Geometry check sheet. Reference: the model listing, model coordinates, mm. Face numbers are marked on the shaded views. A direction names the side the tool comes from. Coordinates: 2 decimals unless noted, no trailing zeros. Write each loop counter-clockwise with the first axis right and the second up, starting at its lowest first coordinate (ties: lowest second). Pieces come first, ordered by that corner, then holes. Notation, with made-up numbers: (88, 37.5) -> (112, 37.5) arc R27 ccw to (112, 72.5) -> close; hole circle Ø6 at (83.5, 38). An arc over 180 degrees is marked (long way). Use a Markdown table: item, result.
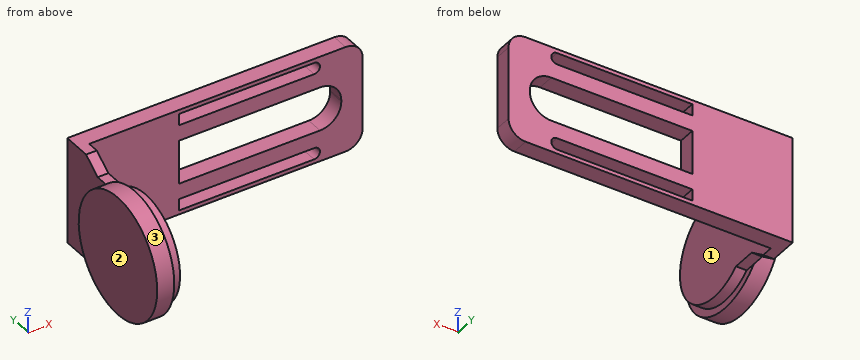
```python
from build123d import *

# Parameters (mm, degrees)
BOSS_EXTRUDE1_DEPTH = 4
BOSS_EXTRUDE2_DEPTH = 2.5
SKETCH3_R           = 14
BOSS_EXTRUDE3_DEPTH = 4


with BuildPart() as part:
    # Sketch1 → Boss-Extrude1 (new body)
    with BuildSketch(Plane(origin=(0, 0, 0), x_dir=(1, 0, 0), z_dir=(0, 1, 0))):
        with BuildLine():
            Line((0, 0), (62.5, 0))
            ThreePointArc((62.5, 0), (65.328427125, -1.171572875), (66.5, -4))
            Line((66.5, -4), (66.5, -21))
            ThreePointArc((66.5, -21), (65.328427125, -23.828427125), (62.5, -25))
            Line((62.5, -25), (0, -25))
            Line((0, -25), (0, 0))
        make_face()
        with BuildLine():
            Line((23.5, -7.35), (56.51, -7.35))
            ThreePointArc((56.51, -7.35), (60.038462838, -8.811537162), (61.5, -12.34))
            Line((61.5, -12.34), (61.5, -12.66))
            ThreePointArc((61.5, -12.66), (60.038462838, -16.188462838), (56.51, -17.65))
            Line((56.51, -17.65), (23.5, -17.65))
            Line((23.5, -17.65), (23.5, -7.35))
        make_face(mode=Mode.SUBTRACT)
        with BuildLine():
            Line((23.5, -0.96), (55.151, -0.96))
            ThreePointArc((55.151, -0.96), (56.104887048, -1.355112952), (56.5, -2.309))
            Line((56.5, -2.309), (56.5, -2.311))
            ThreePointArc((56.5, -2.311), (56.104887048, -3.264887048), (55.151, -3.66))
            Line((55.151, -3.66), (23.5, -3.66))
            Line((23.5, -3.66), (23.5, -0.96))
        make_face(mode=Mode.SUBTRACT)
        with BuildLine():
            Line((23.5, -21.34), (55.151, -21.34))
            ThreePointArc((55.151, -21.34), (56.104887048, -21.735112952), (56.5, -22.689))
            Line((56.5, -22.689), (56.5, -22.691))
            ThreePointArc((56.5, -22.691), (56.104887048, -23.644887048), (55.151, -24.04))
            Line((55.151, -24.04), (23.5, -24.04))
            Line((23.5, -24.04), (23.5, -21.34))
        make_face(mode=Mode.SUBTRACT)
    extrude(amount=BOSS_EXTRUDE1_DEPTH)

    # Sketch2 → Boss-Extrude2 (add)
    with BuildSketch(Plane.ZY):
        with BuildLine():
            Line((3, -6.816145851), (3, -12.416145851))
            ThreePointArc((3, -12.416145851), (12.5, -32.4), (22, -12.416145851))
            Line((22, -12.416145851), (22, -6.816145851))
            Line((22, -6.816145851), (25, -2.7))
            Line((25, -2.7), (25, 0))
            Line((25, 0), (0, 0))
            Line((0, 0), (0, -2.7))
            Line((0, -2.7), (3, -6.816145851))
        make_face()
    extrude(amount=-BOSS_EXTRUDE2_DEPTH)

    # Sketch3 → Boss-Extrude3 (add)
    with BuildSketch(Plane.ZY):
        with Locations(Location((12.5, -20.15, 0), (0, 0, 132.732110043))):
            Circle(SKETCH3_R)
    extrude(amount=BOSS_EXTRUDE3_DEPTH)


solid = part.part
```
Item 1: Section check C-C on y = -20.15. Record the boundary of the cut face in (x, z), then the cut area to 3 significant figures.
Answer block:
| item | result |
|---|---|
| outline | (-4, -1.5) -> (0, -1.5) -> (0, 0.25) -> (2.5, 0.25) -> (2.5, 24.75) -> (0, 24.75) -> (0, 26.5) -> (-4, 26.5) -> close |
| area | 173 mm^2 |
Item 2: Section check D-D on z = 19. Record the boundary of the cut face in (x, y), then the cut area to 3 significant figures.
Answer block:
| item | result |
|---|---|
| outline | (-4, -32.55) -> (0, -32.55) -> (0, -30.53) -> (2.5, -30.53) -> (2.5, 0) -> (66.5, 0) -> (66.5, 4) -> (0, 4) -> (0, -7.75) -> (-4, -7.75) -> close |
| area | 442 mm^2 |
Item 3: Tool access check on the marked faces 1, 2 and 3. Record the directions out of +Z, -Z, +X, -X, +Y, -Y that give a thin tool (end or side, any length) a straight path to the whole face; none if there is none.
Answer block:
| item | result |
|---|---|
| face 1 | +Z, -Z, +X, -Y |
| face 2 | +Z, -Z, -X, +Y, -Y |
| face 3 | -X |
Item 4: Section check B-B on z = 15. Record the boundary of the cut face in (x, y), then the cut area to 3 significant figures.
Answer block:
| item | result |
|---|---|
| outline | (-4, -33.92) -> (0, -33.92) -> (0, -32.14) -> (2.5, -32.14) -> (2.5, 0) -> (23.5, 0) -> (23.5, 4) -> (0, 4) -> (0, -6.38) -> (-4, -6.38) -> close; (60.92, 0) -> (66.5, 0) -> (66.5, 4) -> (60.92, 4) -> close |
| area | 307 mm^2 |
Item 5: Section check A-A on x = 28. Record the boundary of the cut face in (y, z).
Answer block:
| item | result |
|---|---|
| outline | (0, 0) -> (4, 0) -> (4, 0.96) -> (0, 0.96) -> close; (0, 3.66) -> (4, 3.66) -> (4, 7.35) -> (0, 7.35) -> close; (0, 17.65) -> (4, 17.65) -> (4, 21.34) -> (0, 21.34) -> close; (0, 24.04) -> (4, 24.04) -> (4, 25) -> (0, 25) -> close |
Item 6: Thickness scan on L1, parallel to X at y = -26.5, z = 6.5; L2, parallel to X at y = -3, z = 7.5; L3, parallel to Y at x = 21.5, z = 12.25. Record the ranges inside material, lowest first. Write a range as [from, to].
Answer block:
| item | result |
|---|---|
| L1 | x = [-4, 2.5] |
| L2 | x = [0, 2.5] |
| L3 | y = [0, 4] |
Item 7: Depth check by flat-ended pin: P1, Ø1.5, axis at y = -1, z = 16.5, coming from the -X side; P2, Ø1.2, axis at x = 39, y = 3, coming from the +Z side; P3, Ø1.3, axis at y = 3, z = 22.5, coming from the +X side. Enter the tip coordinate at first touch or a pass-through.
Answer block:
| item | result |
|---|---|
| P1 | stops at x = 0 |
| P2 | stops at z = 25 |
| P3 | stops at x = 66.41 |
